Here's how the part is built. I have some questions about the finished solid (model axes, mm). Face numbers are marked on the shaded views. A direction names the side the tool comes from. Round coordinates to 2 decimals unless told otherwise and drop trailing zeros. Order: outer loops, then holes, each group sorted by start corner. A loop starts at its lowest first (then second) coordinate and runs counter-clockwise, first axis right, second up. Notation, with made-up numbers: (58, -21.75) -> (85, -21.75) arc R19 cw to (85, 5.25) -> close; hole circle Ø3 at (46, 36.5). An arc over 180 degrees is marked (long way). Answer in a Markdown table with one row per item.
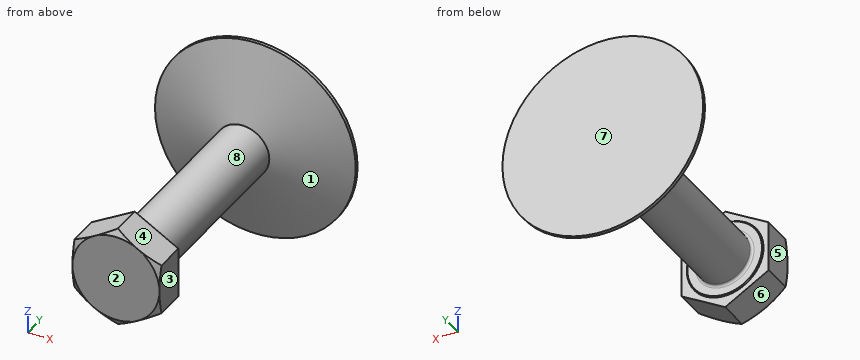
Solid Edge part; units mm, degrees
sketch "Sketch1" plane through (0, 0, 0) normal (0, -1, 0) x (1, 0, 0)
  line L0 (6.5, -3.7528) -> (6.5, 3.7528)
  line L1 (6.5, 3.7528) -> (0, 7.5056)
  line L2 (0, 7.5056) -> (-6.5, 3.7528)
  line L3 (-6.5, 3.7528) -> (-6.5, -3.7528)
  line L4 (-6.5, -3.7528) -> (0, -7.5056)
  line L5 (0, -7.5056) -> (6.5, -3.7528)
extrude "Protrusion1" add sketch "Sketch1" along normal blind 5.3
sketch "Sketch2" plane through (0, 0, 0) normal (1, 0, 0) x (0, 1, 0)
  line L0 (-5.3, 6.5) -> (-4.7194, 7.5056)
revolve "RevolvedCutout1" cut sketch "Sketch2" angle 360 about axis through (0, 0, 0) along (0, -1, 0) material side at (0, -5.053, 7.0278)
sketch "Sketch3" plane through (0, 0, 0) normal (0, 1, 0) x (0.866, 0, -0.5)
  circle A0 centre (0, 0) radius 5.735
extrude "拉伸除料_1" cut sketch "Sketch3" against normal blind 0.15 flip side to cut
sketch "Sketch4" plane through (0, 0, 0) normal (0, 1, 0) x (0, 0, -1)
  circle A0 centre (0, 0) radius 4
extrude "拉伸_2" add sketch "Sketch4" along normal blind 30
chamfer "倒斜角_1" distance 0.8 angle 45 1 edges at (0, 30, 4)
fillet "倒圆_1" radius 0.4 1 edges at (0, 0, 4)
chamfer "倒斜角_2" distance 0.15 angle 45 1 edges at (-4.9667, 0, 2.8675)
cosmetic_thread "Thread1"
sketch "Sketch5" plane through (0, 0, 0) normal (0, 0, 1) x (1, 0, 0)
  line L0 (0, 33.2) -> (15, 33.2)
  line L1 (15, 33.2) -> (15, 32.7)
  line L2 (15, 32.7) -> (4, 29.2)
  line L3 (4, 29.2) -> (0, 29.2)
revolve "RevolvedProtrusion1" add sketch "Sketch5" angle 360 about axis through (0, 29.2, 0) along (0, 1, 0)
1. Suppose I cut it at A-A on y = 24.5. Write out the boundary of the cut face in (x, z).
Numbers:
| item | result |
|---|---|
| outline | circle Ø8 at (0, 0) |
2. For pin 1 Ø2.5 at (y, z) = (-2, 0) entering from -X; pin 2 Ø5 at (x, y) = (-4.5, 20.5) entering from +Z, each with a flat end and sliding along its axis, tell me the tip position at first contact or that it passes through.
Numbers:
| item | result |
|---|---|
| pin 1 | stops at x = -6.5 |
| pin 2 | stops at z = 3.46 |
3. We'd pull the mould along Y, two halves only. Please class the marked faces 1, 2 and 3: released by +Y, released by -Y, zero draft, split by the parting line, or undercut.
Numbers:
| item | result |
|---|---|
| face 1 | undercut |
| face 2 | released by -Y |
| face 3 | zero draft |
4. Please list where these lines run through material, in increasing order: line 1 along Z through (x, y) = (0.25, 20.5); line 2 along Y through (x, z) = (2.25, 3.5); line 3 along Y through (x, z) = (9, 1.5).
Numbers:
| item | result |
|---|---|
| line 1 | z = -3.99 to 3.99 |
| line 2 | y = -5.3 to 0.08, 29.25 to 33.2 |
| line 3 | y = 30.83 to 33.2 |
5. For the marked faces 4, 5, 6, 7 and 8, which set-ups out of +Z, -Z, +X, -X, +Y, -Y let a thin tool reach every point of the face, with its end or its side?
Numbers:
| item | result |
|---|---|
| face 4 | +Z, +X, -Y |
| face 5 | +Z, -Z, -X, -Y |
| face 6 | -Z, -X, -Y |
| face 7 | +Z, -Z, +X, -X, +Y |
| face 8 | none |
